Geometry: final body of the model. Coordinates: model frame, mm. Coordinates: 2 decimals unless noted, no trailing zeros. Order: outer loops, then holes, each group sorted by start corner. A loop starts at its lowest first (then second) coordinate and runs counter-clockwise, first axis right, second up. Notation, with made-up numbers: (62, -14.75) -> (110, -14.75) arc R17 ccw to (110, 13.25) -> close; hole circle Ø6 at (7, 61.5). An arc over 180 degrees is marked (long way). Use one line per item in the form item = value.
```python
from build123d import *

# Parameters (mm, degrees)
BOSS_EXTRUDE1_DEPTH = 15.621


with BuildPart() as part:
    # Sketch1 → Boss-Extrude1 (new body)
    with BuildSketch(Plane.XY):
        with BuildLine():
            Line((-7.005505105, 0), (7.005505105, 0))
            ThreePointArc((7.005505105, 0), (7.764711356, -0.759206251), (7.005505105, -1.518412501))
            Line((7.005505105, -1.518412501), (-7.005505105, -1.518412501))
            ThreePointArc((-7.005505105, -1.518412501), (-7.666300268, -2.179207663), (-7.005505105, -2.840002826))
            Line((-7.005505105, -2.840002826), (7.005505105, -2.840002826))
            Line((7.005505105, -2.840002826), (7.005505105, -3.221002826))
            Line((7.005505105, -3.221002826), (-7.005505105, -3.221002826))
            ThreePointArc((-7.005505105, -3.221002826), (-8.047300268, -2.179207663), (-7.005505105, -1.137412501))
            Line((-7.005505105, -1.137412501), (7.005505105, -1.137412501))
            ThreePointArc((7.005505105, -1.137412501), (7.383711356, -0.759206251), (7.005505105, -0.381))
            Line((7.005505105, -0.381), (-7.005505105, -0.381))
            ThreePointArc((-7.005505105, -0.381), (-8.047300268, 0.660795162), (-7.005505105, 1.702590324))
            Line((-7.005505105, 1.702590324), (7.005505105, 1.702590324))
            ThreePointArc((7.005505105, 1.702590324), (7.528208531, 2.225293749), (7.005505105, 2.747997174))
            Line((7.005505105, 2.747997174), (-7.005505105, 2.747997174))
            Line((-7.005505105, 2.747997174), (-7.005505105, 3.128997174))
            Line((-7.005505105, 3.128997174), (7.005505105, 3.128997174))
            ThreePointArc((7.005505105, 3.128997174), (7.909208531, 2.225293749), (7.005505105, 1.321590324))
            Line((7.005505105, 1.321590324), (-7.005505105, 1.321590324))
            ThreePointArc((-7.005505105, 1.321590324), (-7.666300268, 0.660795162), (-7.005505105, 0))
        make_face()
    extrude(amount=BOSS_EXTRUDE1_DEPTH)


solid = part.part
```
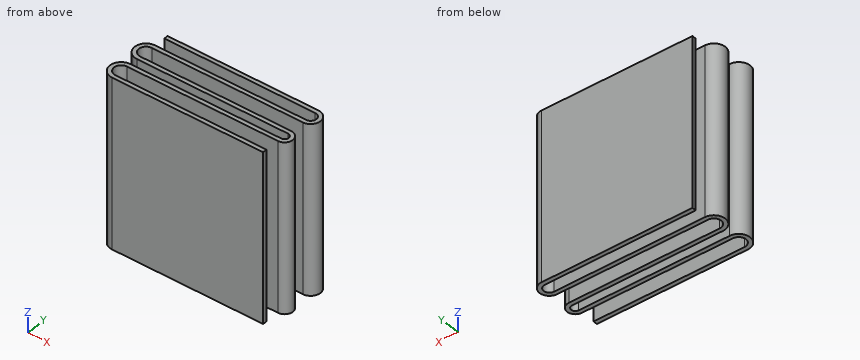
1) Section C-C, the plane y = -2.5. Output: boundary loops of the cut face in (x, z), and give its area (3 significant figures).
Results found:
outline = (-8, 0) -> (-7.58, 0) -> (-7.58, 15.62) -> (-8, 15.62) -> close
area = 6.46 mm2
2) Section B-B, the plane z = 12.5. Output: boundary loops of the cut face in (x, y).
Results found:
outline = (-7.01, -3.22) -> (7.01, -3.22) -> (7.01, -2.84) -> (-7.01, -2.84) arc R0.66 cw to (-7.01, -1.52) -> (7.01, -1.52) arc R0.76 ccw to (7.01, 0) -> (-7.01, 0) arc R0.66 cw to (-7.01, 1.32) -> (7.01, 1.32) arc R0.9 ccw to (7.01, 3.13) -> (-7.01, 3.13) -> (-7.01, 2.75) -> (7.01, 2.75) arc R0.52 cw to (7.01, 1.7) -> (-7.01, 1.7) arc R1.04 ccw to (-7.01, -0.38) -> (7.01, -0.38) arc R0.38 cw to (7.01, -1.14) -> (-7.01, -1.14) arc R1.04 ccw to start
3) Material intervals for probe 1 along Y at (x, z) = (-1.5, 9); probe 2 along X at (y, z) = (-0.75, 3.5); probe 3 along X at (y, z) = (1.5, 8.75), sorted ascending. Write a range as from..to.
Results found:
probe_1 = -3.22..-2.84, -1.52..-1.14, -0.38..0, 1.32..1.7, 2.75..3.13
probe_2 = 7.38..7.76
probe_3 = -7.62..7.54
4) Contact query for a flat-ended pin moving along its axis: P1, Ø2, axis at y = 0.5, z = 8, coming from the -X side. Output: stop coordinate, or through.
Results found:
P1 = -8.05
5) Section A-A, the plane x = 6. Output: boundary loops of the cut face in (y, z).
Results found:
outline = (-3.22, 0) -> (-2.84, 0) -> (-2.84, 15.62) -> (-3.22, 15.62) -> close; (-1.52, 0) -> (-1.14, 0) -> (-1.14, 15.62) -> (-1.52, 15.62) -> close; (-0.38, 0) -> (0, 0) -> (0, 15.62) -> (-0.38, 15.62) -> close; (1.32, 0) -> (1.7, 0) -> (1.7, 15.62) -> (1.32, 15.62) -> close; (2.75, 0) -> (3.13, 0) -> (3.13, 15.62) -> (2.75, 15.62) -> close
